```python
from build123d import *

# Parameters (mm, degrees)
F1_DEPTH = 27
F2_R     = 4
F3_DEPTH = 2
F4_R     = 4
F5_DEPTH = 5
F6_R     = 1


with BuildPart() as f1:
    # F0 (on Top) → F1 (new body)
    with BuildSketch(Plane.XY):
        Polygon((5.196152, 9), (-5.196152, 9), (-10.392305, 0), (-5.196152, -9), (5.196152, -9), (10.392305, 0), align=None)
        Polygon((-8.082904, 0), (-4.041452, 7), (4.041452, 7), (8.082904, 0), (4.041452, -7), (-4.041452, -7), align=None, mode=Mode.SUBTRACT)
    extrude(amount=F1_DEPTH)

    # F2 (on face) → F3 (join)
    with BuildSketch(Plane.XY.offset(27)):
        Polygon((5.196152, 9), (-5.196152, 9), (-10.392305, 0), (-5.196152, -9), (5.196152, -9), (10.392305, 0), align=None)
        Circle(F2_R, mode=Mode.SUBTRACT)
    extrude(amount=-F3_DEPTH)

    # F4 (on face) → F5 (join)
    with BuildSketch(Plane.XY.offset(27)):
        Polygon((3.954849, 6.85), (-3.954849, 6.85), (-7.909699, 0), (-3.954849, -6.85), (3.954849, -6.85), (7.909699, 0), align=None)
        Circle(F4_R, mode=Mode.SUBTRACT)
    extrude(amount=F5_DEPTH)

    # F6
    f6_edges = [f1.edges().sort_by_distance(p)[0] for p in [
        (0, 6.85, 32),
        (-5.932274, 3.425, 32),
        (-5.932274, -3.425, 32),
        (0, -6.85, 32),
        (5.932274, -3.425, 32),
        (5.932274, 3.425, 32),
    ]]
    fillet(f6_edges, radius=F6_R)


solid = f1.part
```
CAD build for the part. Positions are in the model's coordinates, mm. A direction names the side the tool comes from. Coordinates: 2 decimals unless noted, no trailing zeros. Loops run counter-clockwise (first coordinate to the right, second up) from the corner with the lowest first, then second, coordinate; pieces in that order, holes last. Notation, with made-up numbers: (83, -21) - (113, -21) arc R16 cw to (113, -10) - close; hole circle Ø9 at (-26.75, 84). An arc over 180 degrees is marked (long way). Return JSON: item names as keys, results as strings.
1. Drop flat-ended pins along their axis: pin 1 (7 mm diameter, centred on x = -2.5, y = 0, fed in from -Z); pin 2 (3 mm diameter, centred on y = 4.5, z = 28, fed in from -X); pin 3 (1.2 mm diameter, centred on x = 1, z = 28.5, fed in from -Y); pin 4 (7 mm diameter, centred on x = 0, y = 0, fed in from +Z). Give the stop position or say it passes through.
Result:
{"pin 1": "stops at z = 25", "pin 2": "stops at x = -8.44", "pin 3": "stops at y = -6.85", "pin 4": "passes through"}
2. Mould opens along Y. For faces 4 (the flat face through (-6.09, 3.45, 12.32)), 5 (the cylindrical face through (-5.7, 3.227, 31.715)), 6 (the flat face through (5.905, -3.473, 28.972)) say: released by +Y, released by -Y, zero draft, split by the parting line, or undercut.
Result:
{"face 4": "undercut", "face 5": "released by +Y", "face 6": "released by -Y"}
3. 3-axis set-ups, long thin cutter, end or side, ignore diameter. For faces 1 (the flat face through (0, -6.85, 29)), 2 (the flat face through (0, 7, 12)), 3 (the flat face through (-5.905, 3.473, 28.972)): which of +Z, -Z, +X, -X, +Y, -Y reach the whole face in a straight line?
Result:
{"face 1": "+Z, +X, -X, -Y", "face 2": "-Z", "face 3": "+Z, -X, +Y"}
4. Probe L1, parallel to Y at x = 0, z = 14.5; L2, parallel to Y at x = 0, z = 27.75; L3, parallel to Z at x = -0.5, y = 5.75. List the from-to ranges inside material, lowest first. Write a range as from..to.
Result:
{"L1": "y = -9..-7, 7..9", "L2": "y = -6.85..-4, 4..6.85", "L3": "z = 25..32"}
5. Band-saw the part on B-B (z = 20). Give the cut face in (x, y), and give its area (3 significant figures).
Result:
{"outline": "(-10.39, 0) - (-5.2, -9) - (5.2, -9) - (10.39, 0) - (5.2, 9) - (-5.2, 9) - close; hole (-8.08, 0) - (-4.04, -7) - (4.04, -7) - (8.08, 0) - (4.04, 7) - (-4.04, 7) - close", "area": "111 mm2"}
6. Band-saw the part on A-A (x = 0). Give the cut face in (y, z), and give its area (3 significant figures).
Result:
{"outline": "(-9, 0) - (-7, 0) - (-7, 25) - (-4, 25) - (-4, 32) - (-5.85, 32) arc R1 ccw to (-6.85, 31) - (-6.85, 27) - (-9, 27) - close; (4, 25) - (7, 25) - (7, 0) - (9, 0) - (9, 27) - (6.85, 27) - (6.85, 31) arc R1 ccw to (5.85, 32) - (4, 32) - close", "area": "148 mm2"}
